Here's how the part is built. I have some questions about the finished solid (model axes, mm). A direction names the side the tool comes from. Give positions to 0.01 mm unless a question says otherwise; leave off trailing zeros. Loops run counter-clockwise (first coordinate to the right, second up) from the corner with the lowest first, then second, coordinate; pieces in that order, holes last.
Q1. I'm going to push flat-ended pins straight in: P1, Ø0.9, axis at x = -15.5, y = 4, coming from the -Z side; P2, Ø2, axis at x = -1.5, y = 5.5, coming from the -Z side. Where does each tip first touch, or does it pass through?
Q2. I need wall thicknesses on probe 1 along Y at (x, z) = (11.5, -20); probe 2 along X at (y, z) = (-4.5, -11.5); probe 3 along Y at (x, z) = (15.5, -7). Which ranges of each line are inside material? Lowest first, please.
Q3. Suppose I cut it at D-D (x = -5). List the corners of the cut face in (y, z) for me, and give its area (3 significant figures).
Q4. Suppose I cut it at C-C (y = 4.75). List the corners of the cut face in (x, z) for me, and give its area (4 significant figures).
Q5. Suppose I cut it at A-A (z = -3.5). List the corners of the cut face in (x, y) for me, and give its area (3 significant figures).
Q6. Thinking about a two-plate mould opening in Z: for faces 1 (the face through (-0.23, -9.76, -21.99)), 2 (the face through (13, -6.3, -7)), 3 (the face through (-15, 4, -15)), which applies, pulls with the +Z half, pulls with the -Z half, needs draft (parallel to the pull), parting line crosses it, or undercut?
Q7. For faces 4 (the face through (0, 0, 0)), 5 (the face through (9.75, 0, -7)), 6 (the face through (-0.23, 9.74, -22.01)), 7 (the face through (-15, -2.02, -7)), which set-ups out of +Z, -Z, +X, -X, +Y, -Y let a thin tool reach every point of the face, with its end or its side?
Q8. Suppose I cut it at B-B (z = -19.75). List the corners of the cut face in (x, y) for me, and give its area (3 significant figures).
```python
from build123d import *

# Parameters (mm, degrees)
SKETCH1_W           = 32.5
SKETCH1_H           = 26.5
BOSS_EXTRUDE1_DEPTH = 4
SKETCH2_W           = 6.5
SKETCH2_H           = 6.3
BOSS_EXTRUDE2_DEPTH = 15
SKETCH3_W           = 32.5
SKETCH3_H           = 3
BOSS_EXTRUDE3_DEPTH = 22.5
SKETCH4_W           = 32.5
SKETCH4_H           = 1
BOSS_EXTRUDE4_DEPTH = 1
CUT_EXTRUDE1_DEPTH  = 33.5
SKETCH6_W           = 32.5
SKETCH6_H           = 1
BOSS_EXTRUDE5_DEPTH = 1
CUT_EXTRUDE2_DEPTH  = 33.5
SKETCH8_W           = 3
SKETCH8_H           = 3.5
BOSS_EXTRUDE6_DEPTH = 15


with BuildPart() as part:
    # Sketch1 → Boss-Extrude1 (new body)
    with BuildSketch(Plane.XY):
        Rectangle(SKETCH1_W, SKETCH1_H)
    extrude(amount=BOSS_EXTRUDE1_DEPTH)

    # Sketch2 → Boss-Extrude2 (add)
    with BuildSketch(Plane(origin=(0, 0, 0), x_dir=(-1, 0, 0), z_dir=(0, 0, -1))):
        with Locations((-13, -3.15)):
            Rectangle(SKETCH2_W, SKETCH2_H)
        with Locations((-13, 3.15)):
            Rectangle(SKETCH2_W, SKETCH2_H)
    extrude(amount=BOSS_EXTRUDE2_DEPTH)

    # Sketch3 → Boss-Extrude3 (add)
    with BuildSketch(Plane(origin=(0, 0, 0), x_dir=(-1, 0, 0), z_dir=(0, 0, -1))):
        with Locations((0, -11.75)):
            Rectangle(SKETCH3_W, SKETCH3_H)
        with Locations((0, 11.75)):
            Rectangle(SKETCH3_W, SKETCH3_H)
    extrude(amount=BOSS_EXTRUDE3_DEPTH)

    # Sketch4 → Boss-Extrude4 (add)
    with BuildSketch(Plane(origin=(0, -10.25, 0), x_dir=(1, 0, 0), z_dir=(0, 1, 0))):
        with Locations((0, 22)):
            Rectangle(SKETCH4_W, SKETCH4_H)
    extrude(amount=BOSS_EXTRUDE4_DEPTH)

    # Sketch5 → Cut-Extrude1 (cut, through all)
    with BuildSketch(Plane.ZY.offset(16.25)):
        Polygon((-21.5, -10.25), (-22.5, -9.25), (-21.5, -9.25), align=None)
    extrude(amount=-CUT_EXTRUDE1_DEPTH, mode=Mode.SUBTRACT)

    # Sketch6 → Boss-Extrude5 (add)
    with BuildSketch(Plane.XZ.offset(-10.25)):
        with Locations((0, -22)):
            Rectangle(SKETCH6_W, SKETCH6_H)
    extrude(amount=BOSS_EXTRUDE5_DEPTH)

    # Sketch7 → Cut-Extrude2 (cut, through all)
    with BuildSketch(Plane.ZY.offset(16.25)):
        Polygon((-21.5, 10.25), (-21.5, 9.25), (-22.5, 9.25), align=None)
    extrude(amount=-CUT_EXTRUDE2_DEPTH, mode=Mode.SUBTRACT)

    # Sketch8 → Boss-Extrude6 (add)
    with BuildSketch(Plane(origin=(0, 0, 0), x_dir=(-1, 0, 0), z_dir=(0, 0, -1))):
        with Locations((14.75, 3.75)):
            Rectangle(SKETCH8_W, SKETCH8_H)
        with Locations((14.75, -3.76990678)):
            Rectangle(SKETCH8_W, SKETCH8_H)
    extrude(amount=BOSS_EXTRUDE6_DEPTH)


solid = part.part
```
Solutions:
1. P1: stops at z = -15
1. P2: stops at z = 0
2. probe 1: y = -13.25 to -10.25, 10.25 to 13.25
2. probe 2: x = -16.25 to -13.25, 9.75 to 16.25
2. probe 3: y = -13.25 to -10.25, -6.3 to 6.3, 10.25 to 13.25
3. outline: (-13.25, -22.5) - (-9.25, -22.5) - (-10.25, -21.5) - (-10.25, 0) - (10.25, 0) - (10.25, -21.5) - (9.25, -22.5) - (13.25, -22.5) - (13.25, 4) - (-13.25, 4) - close
3. area: 242 mm2
4. outline: (-16.25, -15) - (-13.25, -15) - (-13.25, 0) - (9.75, 0) - (9.75, -15) - (16.25, -15) - (16.25, 4) - (-16.25, 4) - close
4. area: 272.5 mm2
5. outline: (-16.25, -13.25) - (16.25, -13.25) - (16.25, -10.25) - (-16.25, -10.25) - close; (-16.25, -5.52) - (-13.25, -5.52) - (-13.25, -2.02) - (-16.25, -2.02) - close; (-16.25, 2) - (-13.25, 2) - (-13.25, 5.5) - (-16.25, 5.5) - close; (-16.25, 10.25) - (16.25, 10.25) - (16.25, 13.25) - (-16.25, 13.25) - close; (9.75, -6.3) - (16.25, -6.3) - (16.25, 6.3) - (9.75, 6.3) - close
5. area: 298 mm2
6. face 1: undercut
6. face 2: needs draft
6. face 3: pulls with the -Z half
7. face 4: none
7. face 5: -Z
7. face 6: +X, -X
7. face 7: -Z, -X
8. outline: (-16.25, -13.25) - (16.25, -13.25) - (16.25, -10.25) - (-16.25, -10.25) - close; (-16.25, 10.25) - (16.25, 10.25) - (16.25, 13.25) - (-16.25, 13.25) - close
8. area: 195 mm2
